CAD build for the part. Positions are in the model's coordinates, mm. Coordinates: 2 decimals unless noted, no trailing zeros. Loops run counter-clockwise (first coordinate to the right, second up) from the corner with the lowest first, then second, coordinate; pieces in that order, holes last. Notation, with made-up numbers: (-6.5, -31.75) -> (36.5, -31.75) arc R10 cw to (36.5, -17.75) -> close; hole circle Ø10 at (53.5, 38.25). An arc over 180 degrees is marked (long way). Return JSON: item names as keys, results as strings. Group by question number.
(1) Saw through at B-B on y = 7.75. Give the number of separate pieces and of enclosed holes in the cut face, then the cut area to 3 significant figures.
(2) Probe L1, parallel to X at y = 2.5, z = -6; L2, parallel to X at y = 7.5, z = 62.5 (3 decimals); L3, parallel to Y at x = -87, z = 29. List the from-to ranges inside material, lowest first.
(3) Flat gauge pins, fed straight in: pin 1 Ø15 at (x, z) = (-76, 31) entering from +Y; pin 2 Ø5 at (y, z) = (17, 64) entering from -X; pin 3 Ø14.5 at (y, z) = (19, 73) entering from -X; pin 4 Ø9 at (y, z) = (20, -70) entering from +X. Where does each tip first touch, or does it go through?
(4) Saw through at A-A on z = -76. Write the cut outline in (x, y) (3 decimals), then the cut area to 3 significant figures.
```python
from build123d import *

# Parameters (mm, degrees)
BOSS_EXTRUDE1_DEPTH      = 3.81
SKETCH2_W                = 1.27
SKETCH2_H                = 38.1
BOSS_EXTRUDE2_DEPTH      = 25.4
FILLET1_R                = 25.4
SKETCH4_R                = 9.525
SKETCH4_R_2              = 3.175
BOSS_EXTRUDE3_DEPTH      = 12.7
CIRPATTERN5_COUNT        = 8
FILLET1_OF_CIRPATTERN5_R = 25.4
SKETCH5_R                = 95.25
SKETCH5_R_2              = 91.44
BOSS_EXTRUDE4_DEPTH      = 3.81
FILLET2_R                = 2.54


with BuildPart() as part:
    # Sketch1 → Boss-Extrude1 (new body)
    with BuildSketch(Plane(origin=(0, 0, 0), x_dir=(1, 0, 0), z_dir=(0, 1, 0))):
        with BuildLine():
            Line((-0.635, 57.15), (-3.257741865, 8.950572213))
            ThreePointArc((-3.257741865, 8.950572213), (0, 9.525), (3.257741865, 8.950572213))
            Line((3.257741865, 8.950572213), (0.635, 57.15))
            Line((0.635, 57.15), (0.635, 95.25))
            Line((0.635, 95.25), (-0.635, 95.25))
            Line((-0.635, 95.25), (-0.635, 57.15))
        make_face()
    boss_extrude1 = extrude(amount=BOSS_EXTRUDE1_DEPTH)

    # Sketch2 → Boss-Extrude2 (add)
    with BuildSketch(Plane(origin=(0, 3.81, 0), x_dir=(1, 0, 0), z_dir=(0, 1, 0))):
        with Locations((0, 76.2)):
            Rectangle(SKETCH2_W, SKETCH2_H)
    boss_extrude2 = extrude(amount=BOSS_EXTRUDE2_DEPTH)

    # Fillet1
    fillet1_edges = [part.edges().sort_by_distance(p)[0] for p in [
        (0, 3.81, -57.15),
    ]]
    fillet(fillet1_edges, radius=FILLET1_R - 0.0001)  # a hair under: the kernel refuses the full size

    # Sketch4 → Boss-Extrude3 (add)
    with BuildSketch(Plane(origin=(0, 0, 0), x_dir=(1, 0, 0), z_dir=(0, 1, 0))):
        with Locations(Location((0, 0, 0), (0, 0, 70))):
            Circle(SKETCH4_R)
        with Locations(Location((0, 0, 0), (0, 0, 270))):
            Circle(SKETCH4_R_2, mode=Mode.SUBTRACT)
    extrude(amount=BOSS_EXTRUDE3_DEPTH)

    # CirPattern5: Boss-Extrude1, Boss-Extrude2 ×8 about axis
    cirpattern5_axis = Axis((0, 0, 0), (0, 1, 0))
    add([boss_extrude1.rotate(cirpattern5_axis, i * 360 / CIRPATTERN5_COUNT) for i in range(1, CIRPATTERN5_COUNT)])
    add([boss_extrude2.rotate(cirpattern5_axis, i * 360 / CIRPATTERN5_COUNT) for i in range(1, CIRPATTERN5_COUNT)])

    # Fillet1 of CirPattern5
    fillet1_of_cirpattern5_edges = [part.edges().sort_by_distance(p)[0] for p in [
        (-40.411152545, 3.81, -40.411152545),
        (-57.15, 3.81, 0),
        (-40.411152545, 3.81, 40.411152545),
        (0, 3.81, 57.15),
        (40.411152545, 3.81, 40.411152545),
        (57.15, 3.81, 0),
        (40.411152545, 3.81, -40.411152545),
    ]]
    fillet(fillet1_of_cirpattern5_edges, radius=FILLET1_OF_CIRPATTERN5_R - 0.0001)  # a hair under: the kernel refuses the full size

    # Sketch5 → Boss-Extrude4 (add)
    with BuildSketch(Plane(origin=(0, 0, 0), x_dir=(1, 0, 0), z_dir=(0, 1, 0))):
        Circle(SKETCH5_R)
        Circle(SKETCH5_R_2, mode=Mode.SUBTRACT)
    extrude(amount=BOSS_EXTRUDE4_DEPTH)

    # Fillet2
    fillet2_edges = [part.edges().sort_by_distance(p)[0] for p in [
        (-3.257741865, 12.7, 8.950572213),
        (0, 12.7, -3.175),
    ]]
    fillet(fillet2_edges, radius=FILLET2_R)


solid = part.part
```
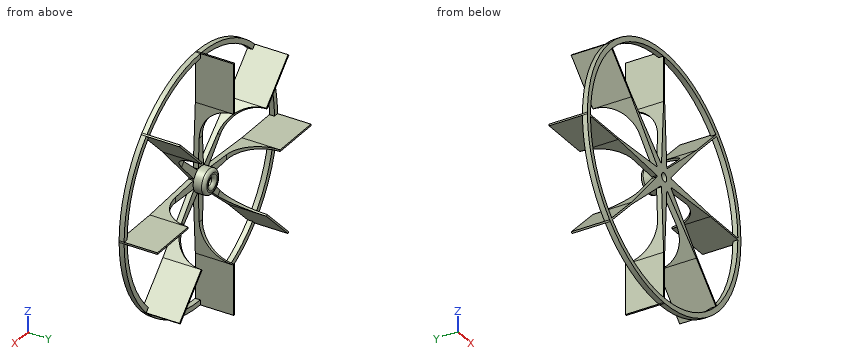
Geometry results:
{
 "1": {"separate pieces": "9", "enclosed holes": "1", "area": "821 mm²"},
 "2": {"L1": "-95.06 to -91.24, -10.4 to 10.4, 91.24 to 95.06", "L2": "-63.398 to -61.602, -0.635 to 0.635, 61.602 to 63.398", "L3": "0 to 3.81"},
 "3": {"pin 1": "through", "pin 2": "x = -67.4", "pin 3": "x = -67.8", "pin 4": "x = 67.8"},
 "4": {"outline": "(-57.416, 0) -> (-50.846, 0) -> (-50.846, 3.81) -> (-57.416, 3.81) -> close; (-0.635, 0) -> (0.635, 0) -> (0.635, 29.21) -> (-0.635, 29.21) -> close; (50.846, 0) -> (57.416, 0) -> (57.416, 3.81) -> (50.846, 3.81) -> close", "area": "87.2 mm²"}
}
